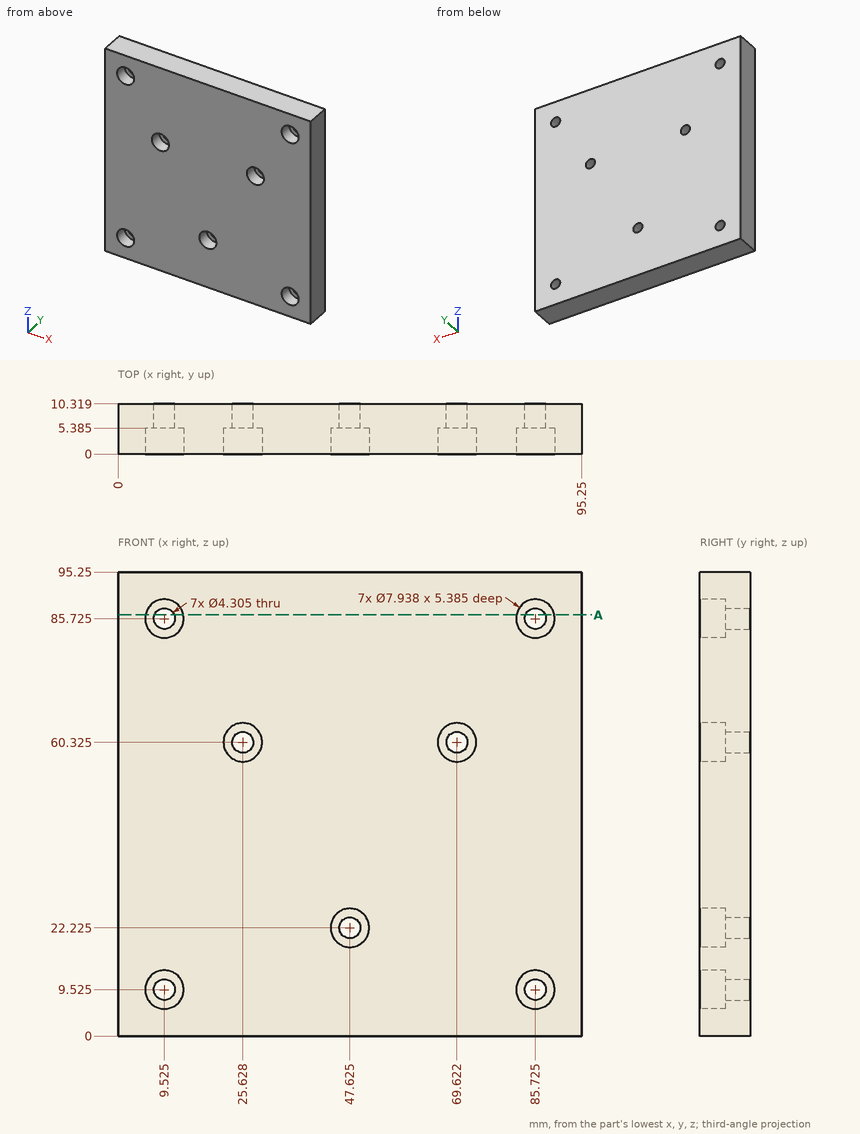
Design review of the part shown in the three views and the two pictorial views. Dimensions are in mm from the part's minimum x, y and z. Round coordinates to 2 decimals unless told otherwise and drop trailing zeros. Use one line per item in the form item = value.
1) Clearance check with flat-ended pins moving along their axes: pin 1 (7 mm diameter, centred on x = 25.63, z = 60.32, fed in from -Y) (1 decimal); pin 2 (8.5 mm diameter, centred on x = 8, z = 86.5, fed in from -Y); pin 3 (4 mm diameter, centred on x = 9.525, z = 9.525, fed in from -Y). State where each tip first meets the part, or that it passes through.
Found:
pin_1 = 5.4
pin_2 = 0
pin_3 = through
2) Take a section at A-A, the plane z = 86.5. Count the separate pieces of the cut face and the enclosed holes in it.
Found:
separate_pieces = 3
enclosed_holes = 0
3) To check wall thickness, follow L1, parallel to X at y = 3, z = 22; L2, parallel to Z at x = 83.5, y = 1; L3, parallel to X at y = 7.75, z = 21.5. State the ranges of each line that lie inside material, in increasing order. Write a range as from..to.
Found:
L1 = 0..43.66, 51.59..95.25
L2 = 0..6.24, 12.81..82.44, 89.01..95.25
L3 = 0..45.6, 49.65..95.25
